Verification items for the finished model (mm, model axes). Face numbers are marked on the shaded views. A direction names the side the tool comes from. Give positions to 0.01 mm unless a question says otherwise; leave off trailing zeros. Order: outer loops, then holes, each group sorted by start corner. A loop starts at its lowest first (then second) coordinate and runs counter-clockwise, first axis right, second up. Notation, with made-up numbers: (37, 76.25) - (94, 76.25) arc R21 cw to (94, 80.25) - close; hole circle Ø10 at (23, 15). An arc over 180 degrees is marked (long way). Answer as a JSON object with one key per item and string values.
```python
from build123d import *

# Parameters (mm, degrees)
F0_R     = 9.525
F1_DEPTH = 12.7
F2_R     = 6.6675
F3_DEPTH = 9.525
F4_R     = 2.59969
F5_DEPTH = 25.4
F6_W     = 1.1938
F6_H     = 2.2352


with BuildPart() as f1:
    # F0 (on Top) → F1 (new body)
    with BuildSketch(Plane.XY):
        Circle(F0_R)
    extrude(amount=F1_DEPTH)

    # F2 (on face) → F3 (cut)
    with BuildSketch(Plane.XY.offset(12.7)):
        Circle(F2_R)
    extrude(amount=-F3_DEPTH, mode=Mode.SUBTRACT)

    # F4 (on face) → F5 (cut)
    with BuildSketch(Plane.XY.offset(3.175)):
        Circle(F4_R)
    extrude(amount=-F5_DEPTH, mode=Mode.SUBTRACT)

    # F6 (on Front) → F7 (revolve, cut)
    with BuildSketch(Plane.XZ):
        with Locations((7.2644, 9.9949)):
            Rectangle(F6_W, F6_H)
    revolve(axis=Axis((0, 0, 19.022157), (0, 0, 1)), mode=Mode.SUBTRACT)


solid = f1.part
```
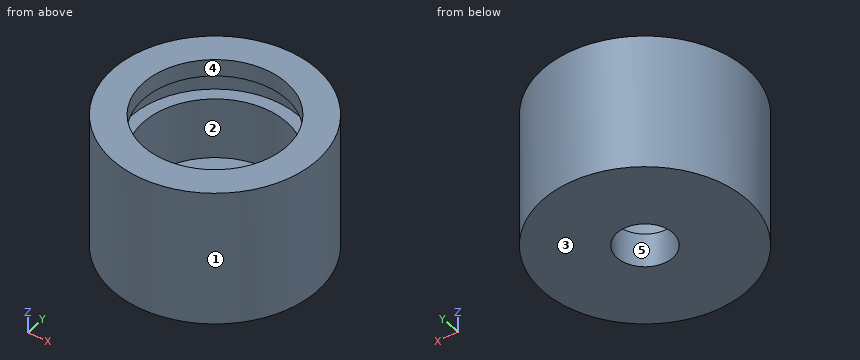
(1) Access from +Z, -Z, +X, -X, +Y, -Y to the whole of each face (thin tool, end or side, straight path). Record for the marked faces 4 and 5.
Computed values:
{"face 4": "+Z", "face 5": "+Z, -Z"}
(2) Release check for a two-part mould opening along Y. For the marked faces 1, 2 and 3 record: pulls with the +Y half, pulls with the -Y half, needs draft (parallel to the pull), parting line crosses it, or undercut.
Computed values:
{"face 1": "parting line crosses it", "face 2": "undercut", "face 3": "needs draft"}
(3) Material ranges on line 1 along Y through (x, z) = (0, 11.5) (1 decimal); line 2 along Z through (x, y) = (-6.75, 2.25); line 3 along X through (y, z) = (0.25, 9), recorded low to high. Write a range as [from, to].
Computed values:
{"line 1": "y = [-9.5, -6.7], [6.7, 9.5]", "line 2": "z = [0, 8.88], [11.11, 12.7]", "line 3": "x = [-9.52, -7.86], [7.86, 9.52]"}
(4) Section check A-A (y = 0). Record the cut outline in (x, z) (1 decimal).
Computed values:
{"outline": "(-9.5, 0) - (-2.6, 0) - (-2.6, 3.2) - (-6.7, 3.2) - (-6.7, 8.9) - (-7.9, 8.9) - (-7.9, 11.1) - (-6.7, 11.1) - (-6.7, 12.7) - (-9.5, 12.7) - close; (2.6, 0) - (9.5, 0) - (9.5, 12.7) - (6.7, 12.7) - (6.7, 11.1) - (7.9, 11.1) - (7.9, 8.9) - (6.7, 8.9) - (6.7, 3.2) - (2.6, 3.2) - close"}
(5) Gauge pin test, flat ends, axial feed: pin 1 Ø4 at (y, z) = (-3, 10) entering from +X; pin 2 Ø1 at (x, z) = (7.5, 8) entering from +Y; pin 3 Ø6.5 at (x, y) = (-1, 0) entering from +Z (3 decimals). Record the tip position at first contact, or that the pin passes through.
Computed values:
{"pin 1": "stops at x = 9.47", "pin 2": "stops at y = 6.46", "pin 3": "stops at z = 3.175"}
(6) Section check D-D (y = 3.75). Record the cut outline in (x, z) (1 decimal).
Computed values:
{"outline": "(-8.8, 0) - (8.8, 0) - (8.8, 12.7) - (5.5, 12.7) - (5.5, 11.1) - (6.9, 11.1) - (6.9, 8.9) - (5.5, 8.9) - (5.5, 3.2) - (-5.5, 3.2) - (-5.5, 8.9) - (-6.9, 8.9) - (-6.9, 11.1) - (-5.5, 11.1) - (-5.5, 12.7) - (-8.8, 12.7) - close"}
(7) Section check C-C (z = 2.5). Record the cut outline in (x, y) (3 decimals), then the cut area to 3 significant figures.
Computed values:
{"outline": "circle Ø19.05 at (0, 0); hole circle Ø5.199 at (0, 0)", "area": "264 mm²"}
